Check sheet for the modelled part. Datum: model origin and axes. Units: mm. Coordinates: 2 decimals unless noted, no trailing zeros. Loops run counter-clockwise (first coordinate to the right, second up) from the corner with the lowest first, then second, coordinate; pieces in that order, holes last.
```python
from build123d import *

# Parameters (mm, degrees)
SKETCH_1_W     = 0.64
SKETCH_1_H     = 0.64
CHAMFER_1_SIZE = 0.1


with BuildPart() as part:
    # По траектории1: sweep along a path in Эскиз2
    with BuildLine(Plane.XY) as sweep_1_path:
        Line((0, 0), (0, 9.48))
        ThreePointArc((0, 9.48), (0.146446609, 9.833553391), (0.5, 9.98))
        Line((0.5, 9.98), (4.48, 9.98))
    # Эскиз1 → По траектории1 (sweep)
    with BuildSketch(Plane(origin=(0, 0, 0), x_dir=(1, 0, 0), z_dir=(0, 1, 0))):
        Rectangle(SKETCH_1_W, SKETCH_1_H)
    sweep(path=sweep_1_path.line)

    # Фаска1
    chamfer_1_edges = [part.edges().sort_by_distance(p)[0] for p in [
        (4.48, 9.98, 0.32),
        (4.48, 10.3, 0),
        (4.48, 9.98, -0.32),
        (0, 0, 0.32),
        (-0.32, 0, 0),
        (0, 0, -0.32),
        (0.32, 0, 0),
    ]]
    chamfer(chamfer_1_edges, length=CHAMFER_1_SIZE)


solid = part.part
```
1) Section check C-C on x = 4.05. Enter the section's corners in (y, z), plus the area to 3 significant figures.
Answer sheet:
outline: (9.66, -0.32) - (10.3, -0.32) - (10.3, 0.32) - (9.66, 0.32) - close
area: 0.410 mm2
2) Section check B-B on y = 7.5. Enter the section's corners in (x, z).
Answer sheet:
outline: (-0.32, -0.32) - (0.32, -0.32) - (0.32, 0.32) - (-0.32, 0.32) - close
3) Mould release check, pull along X, two halves, no side actions. Record for faces 1 (the cylindrical face through (-0.09, 10.05, 0)), 2 (the flat face through (0, 7, 0.32)): +X half, -X half, draft (parallel to the pull), parting line (faces both ways), or undercut.
Answer sheet:
face 1: -X half
face 2: draft
4) Section check A-A on z = 0.1. Enter the section's corners in (x, y), plus the area to 3 significant figures.
Answer sheet:
outline: (-0.32, 0.1) - (-0.22, 0) - (0.22, 0) - (0.32, 0.1) - (0.32, 9.48) arc R0.18 cw to (0.5, 9.66) - (4.48, 9.66) - (4.48, 10.2) - (4.38, 10.3) - (0.5, 10.3) arc R0.82 ccw to (-0.32, 9.48) - close
area: 9.10 mm2
5) Scan lines: line 1 (X direction, y = 5, z = -0.15); line 2 (Y direction, x = 3.6, z = -0.2); line 3 (X direction, y = 10, z = 0.2). Record each from-to range of solid material in increasing order.
Answer sheet:
line 1: x = -0.32 to 0.32
line 2: y = 9.66 to 10.3
line 3: x = -0.13 to 4.48
